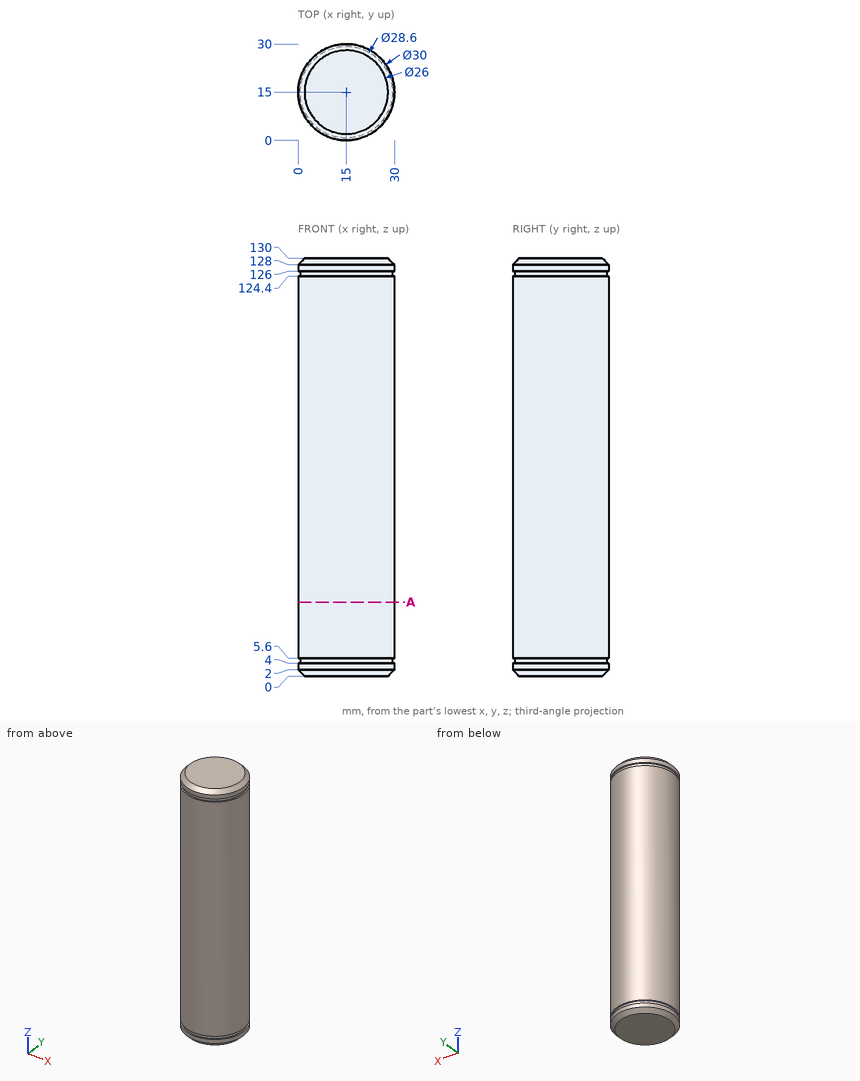
Verification items for this drawing (mm, ordinates from the low corner). Coordinates: 2 decimals unless noted, no trailing zeros. Write each loop counter-clockwise with the first axis right and the second up, starting at its lowest first coordinate (ties: lowest second). Pieces come first, ordered by that corner, then holes. Notation, with made-up numbers: M -9.5,7.5 L 14.5,7.5 A14 cw 14.5,12.5 Z; hole C -4,75 d7. An arc over 180 degrees is marked long. Answer as a JSON object with one key per item and string values.
1. Section check A-A, the plane z = 23. Enter the section's corners in (x, y), plus the area to 3 significant figures.
Answers below:
{"outline": "C 15,15 d30", "area": "707 mm²"}
2. Go/stop test with flat-tipped pins: pin 1 Ø12 at (y, z) = (5.5, 46.5) entering from -X; pin 2 Ø3 at (x, z) = (19, 51) entering from +Y; pin 3 Ø8 at (y, z) = (20.5, 57.5) entering from +X. Record where each tip stops, or that it passes through.
Answers below:
{"pin 1": "stops at x = 0.41", "pin 2": "stops at y = 29.79", "pin 3": "stops at x = 29.92"}
3. Scan lines: L1, parallel to X at y = 14.25, z = 15; L2, parallel to Y at x = 19.5, z = 56; L3, parallel to X at y = 22.5, z = 62. Record each from-to range of solid material in increasing order.
Answers below:
{"L1": "x = 0.02 to 29.98", "L2": "y = 0.69 to 29.31", "L3": "x = 2.01 to 27.99"}
